from build123d import *

# Parameters (mm, degrees)
F1_DEPTH = 5
F2_W     = 5
F2_H     = 5
F3_DEPTH = 85
F4_W     = 2
F4_H     = 10
F5_DEPTH = 5
F6_DEPTH = 5
F7_R     = 1
F8_DEPTH = 10


with BuildPart() as f1:
    # F0 (on Top) → F1 (new body)
    with BuildSketch(Plane.XY):
        Polygon((3.1958913997, 17.8316862418), (3.1958913997, 29.6752474937), (-5.6755073997, 29.6752474937), (-5.6755073997, 17.4481306137), (-3.004598, 19.391063), (-2.590673, 19.643703), (-2.127576, 19.830687), (-1.639877, 19.938255), (-1.14109, 19.963425), (-0.645039, 19.905499), (-0.165471, 19.766083), (0.284322, 19.549041), align=None)
        with BuildLine():
            Line((44.778874, -6.695544), (3.1958913997, 17.8316862418))
            Line((3.1958913997, 17.8316862418), (3.1958913997, 16.96755))
            Line((3.1958913997, 16.96755), (-0.239810875, 16.96755))
            ThreePointArc((-0.239810875, 16.96755), (-1.239808, 15.967552875), (-2.239805125, 16.96755))
            Line((-2.239805125, 16.96755), (-5.6755073997, 16.96755))
            Line((-5.6755073997, 16.96755), (-5.6755073997, 17.4481306137))
            Line((-5.6755073997, 17.4481306137), (-44.778874, -10.997311))
            Line((-44.778874, -10.997311), (-44.506651, -11.416707))
            Line((-44.506651, -11.416707), (-44.230389, -11.833453))
            Line((-44.230389, -11.833453), (-43.950113, -12.24751))
            Line((-43.950113, -12.24751), (-43.66585, -12.65884))
            Line((-43.66585, -12.65884), (-43.377624, -13.067404))
            Line((-43.377624, -13.067404), (-43.085465, -13.473164))
            Line((-43.085465, -13.473164), (-42.789399, -13.876081))
            Line((-42.789399, -13.876081), (-42.489453, -14.276119))
            Line((-42.489453, -14.276119), (-42.185655, -14.673241))
            Line((-42.185655, -14.673241), (-41.878035, -15.067408))
            Line((-41.878035, -15.067408), (-41.56662, -15.458584))
            Line((-41.56662, -15.458584), (-41.25144, -15.846733))
            Line((-41.25144, -15.846733), (-40.932525, -16.231819))
            Line((-40.932525, -16.231819), (-40.609903, -16.613804))
            Line((-40.609903, -16.613804), (-40.283605, -16.992655))
            Line((-40.283605, -16.992655), (-39.953662, -17.368335))
            Line((-39.953662, -17.368335), (-39.620104, -17.74081))
            Line((-39.620104, -17.74081), (-39.282963, -18.110044))
            Line((-39.282963, -18.110044), (-38.942269, -18.476003))
            Line((-38.942269, -18.476003), (-38.598056, -18.838653))
            Line((-38.598056, -18.838653), (-38.250354, -19.19796))
            Line((-38.250354, -19.19796), (-37.899197, -19.553891))
            Line((-37.899197, -19.553891), (-37.544616, -19.906411))
            Line((-37.544616, -19.906411), (-37.486622, -19.963425))
            Line((-37.486622, -19.963425), (-33.507621, -18.914429))
            Line((-33.507621, -18.914429), (-33.877651, -18.578163))
            Line((-33.877651, -18.578163), (-34.244177, -18.23808))
            Line((-34.244177, -18.23808), (-34.60716, -17.894218))
            Line((-34.60716, -17.894218), (-34.966561, -17.546614))
            Line((-34.966561, -17.546614), (-35.322341, -17.195304))
            Line((-35.322341, -17.195304), (-35.674461, -16.840326))
            Line((-35.674461, -16.840326), (-36.022885, -16.481719))
            Line((-36.022885, -16.481719), (-36.367574, -16.119522))
            Line((-36.367574, -16.119522), (-36.708491, -15.753772))
            Line((-36.708491, -15.753772), (-37.045601, -15.384509))
            Line((-37.045601, -15.384509), (-37.378867, -15.011774))
            Line((-37.378867, -15.011774), (-37.708252, -14.635605))
            Line((-37.708252, -14.635605), (-38.033722, -14.256044))
            Line((-38.033722, -14.256044), (-38.355242, -13.87313))
            Line((-38.355242, -13.87313), (-38.672778, -13.486906))
            Line((-38.672778, -13.486906), (-38.986294, -13.097412))
            Line((-38.986294, -13.097412), (-39.295758, -12.704691))
            Line((-39.295758, -12.704691), (-39.601136, -12.308785))
            Line((-39.601136, -12.308785), (-39.902395, -11.909735))
            Line((-39.902395, -11.909735), (-40.199504, -11.507586))
            Line((-40.199504, -11.507586), (-40.262255, -11.421522))
            Line((-40.262255, -11.421522), (-3.665827, 15.200266))
            Line((-3.665827, 15.200266), (-3.339439, 14.822254))
            Line((-3.339439, 14.822254), (-2.954863, 14.503627))
            Line((-2.954863, 14.503627), (-2.522758, 14.253214))
            Line((-2.522758, 14.253214), (-2.055097, 14.077956))
            Line((-2.055097, 14.077956), (-1.564842, 13.982709))
            Line((-1.564842, 13.982709), (-1.06558, 13.970114))
            Line((-1.06558, 13.970114), (-0.571146, 14.040519))
            Line((-0.571146, 14.040519), (-0.095243, 14.191973))
            Line((-0.095243, 14.191973), (0.34894, 14.420279))
            Line((0.34894, 14.420279), (0.749093, 14.719109))
            Line((0.749093, 14.719109), (1.094126, 15.080183))
            Line((1.094126, 15.080183), (1.344177, 15.440914))
            Line((1.344177, 15.440914), (40.323708, -7.550701))
            Line((40.323708, -7.550701), (40.067458, -7.980043))
            Line((40.067458, -7.980043), (39.806774, -8.406706))
            Line((39.806774, -8.406706), (39.541683, -8.830645))
            Line((39.541683, -8.830645), (39.272214, -9.251815))
            Line((39.272214, -9.251815), (38.998395, -9.67017))
            Line((38.998395, -9.67017), (38.720256, -10.085665))
            Line((38.720256, -10.085665), (38.437827, -10.498257))
            Line((38.437827, -10.498257), (38.151138, -10.907899))
            Line((38.151138, -10.907899), (37.86022, -11.31455))
            Line((37.86022, -11.31455), (37.565104, -11.718164))
            Line((37.565104, -11.718164), (37.265821, -12.118698))
            Line((37.265821, -12.118698), (36.962405, -12.51611))
            Line((36.962405, -12.51611), (36.654888, -12.910357))
            Line((36.654888, -12.910357), (36.343302, -13.301397))
            Line((36.343302, -13.301397), (36.02768, -13.689187))
            Line((36.02768, -13.689187), (35.708058, -14.073686))
            Line((35.708058, -14.073686), (35.384469, -14.454852))
            Line((35.384469, -14.454852), (35.056948, -14.832646))
            Line((35.056948, -14.832646), (34.72553, -15.207025))
            Line((34.72553, -15.207025), (34.390251, -15.57795))
            Line((34.390251, -15.57795), (34.318334, -15.656515))
            Line((34.318334, -15.656515), (35.327871, -19.64571))
            Line((35.327871, -19.64571), (35.67992, -19.290661))
            Line((35.67992, -19.290661), (36.028522, -18.932227))
            Line((36.028522, -18.932227), (36.373644, -18.570442))
            Line((36.373644, -18.570442), (36.715254, -18.205338))
            Line((36.715254, -18.205338), (37.05332, -17.836951))
            Line((37.05332, -17.836951), (37.387811, -17.465314))
            Line((37.387811, -17.465314), (37.718695, -17.090462))
            Line((37.718695, -17.090462), (38.045942, -16.712431))
            Line((38.045942, -16.712431), (38.369521, -16.331256))
            Line((38.369521, -16.331256), (38.689401, -15.946971))
            Line((38.689401, -15.946971), (39.005553, -15.559614))
            Line((39.005553, -15.559614), (39.317948, -15.16922))
            Line((39.317948, -15.16922), (39.626556, -14.775825))
            Line((39.626556, -14.775825), (39.931348, -14.379467))
            Line((39.931348, -14.379467), (40.232296, -13.980182))
            Line((40.232296, -13.980182), (40.529372, -13.578008))
            Line((40.529372, -13.578008), (40.822549, -13.172983))
            Line((40.822549, -13.172983), (41.111797, -12.765143))
            Line((41.111797, -12.765143), (41.397092, -12.354527))
            Line((41.397092, -12.354527), (41.678405, -11.941174))
            Line((41.678405, -11.941174), (41.955712, -11.525122))
            Line((41.955712, -11.525122), (42.228985, -11.10641))
            Line((42.228985, -11.10641), (42.498199, -10.685077))
            Line((42.498199, -10.685077), (42.76333, -10.261162))
            Line((42.76333, -10.261162), (43.024353, -9.834706))
            Line((43.024353, -9.834706), (43.281242, -9.405747))
            Line((43.281242, -9.405747), (43.533975, -8.974325))
            Line((43.533975, -8.974325), (43.782527, -8.540482))
            Line((43.782527, -8.540482), (44.026875, -8.104258))
            Line((44.026875, -8.104258), (44.266997, -7.665692))
            Line((44.266997, -7.665692), (44.50287, -7.224827))
            Line((44.50287, -7.224827), (44.734473, -6.781704))
            Line((44.734473, -6.781704), (44.778874, -6.695544))
        make_face()
        with BuildLine():
            Line((3.1958913997, 16.96755), (3.1958913997, 17.8316862418))
            Line((3.1958913997, 17.8316862418), (0.284322, 19.549041))
            Line((0.284322, 19.549041), (-0.165471, 19.766083))
            Line((-0.165471, 19.766083), (-0.645039, 19.905499))
            Line((-0.645039, 19.905499), (-1.14109, 19.963425))
            Line((-1.14109, 19.963425), (-1.639877, 19.938255))
            Line((-1.639877, 19.938255), (-2.127576, 19.830687))
            Line((-2.127576, 19.830687), (-2.590673, 19.643703))
            Line((-2.590673, 19.643703), (-3.004598, 19.391063))
            Line((-3.004598, 19.391063), (-5.6755073997, 17.4481306137))
            Line((-5.6755073997, 17.4481306137), (-5.6755073997, 16.96755))
            Line((-5.6755073997, 16.96755), (-2.239805125, 16.96755))
            ThreePointArc((-2.239805125, 16.96755), (-1.239808, 17.967547125), (-0.239810875, 16.96755))
            Line((-0.239810875, 16.96755), (3.1958913997, 16.96755))
        make_face()
    extrude(amount=F1_DEPTH)

    # F2 (on face) → F3 (join)
    with BuildSketch(Plane(origin=(0, 29.6752474937, 0), x_dir=(-1, 0, 0), z_dir=(0, 1, 0))):
        with Locations((1.239808, 2.5)):
            Rectangle(F2_W, F2_H)
    extrude(amount=F3_DEPTH)

    # F4 (on face) → F5 (join)
    with BuildSketch(Plane.XY.offset(5)):
        with Locations((-4.739808, 109.6752474937)):
            Rectangle(F4_W, F4_H)
        with Locations((2.260192, 109.6752474937)):
            Rectangle(F4_W, F4_H)
    extrude(amount=-F5_DEPTH)

    # F4 (on face) → F6 (cut)
    with BuildSketch(Plane.XY.offset(5)):
        Polygon((-0.239808, 114.6752474937), (-2.239808, 114.6752474937), (-2.739808, 108.6752474937), (0.260192, 108.6752474937), align=None)
    extrude(amount=-F6_DEPTH, mode=Mode.SUBTRACT)

    # F7 (on face) → F8 (cut)
    with BuildSketch(Plane.YZ.offset(3.260192)):
        with Locations((121.0267286794, 2.5)):
            Circle(F7_R)
    extrude(amount=-F8_DEPTH, mode=Mode.SUBTRACT)


solid = f1.part
Verification items for the finished model (mm, model axes). A direction names the side the tool comes from. Coordinates: 2 decimals unless noted, no trailing zeros. Order: outer loops, then holes, each group sorted by start corner. A loop starts at its lowest first (then second) coordinate and runs counter-clockwise, first axis right, second up.
Item 1: Material ranges on L1, parallel to X at y = 18, z = 3.55; L2, parallel to X at y = 82, z = 4.35; L3, parallel to X at y = 11, z = 1.55, recorded low to high.
Filled in:
L1: x = -5.68 to 3.2
L2: x = -3.74 to 1.26
L3: x = -14.54 to -9.44, 8.87 to 14.78
Item 2: Section check B-B, the plane y = 25. Enter the section's corners in (x, z), then the cut area to 3 significant figures.
Filled in:
outline: (-5.68, 0) - (3.2, 0) - (3.2, 5) - (-5.68, 5) - close
area: 44.4 mm2
Item 3: Depth check by flat-ended pin: pin 1 (1.5 mm diameter, centred on y = 74, z = 3.5, fed in from +X); pin 2 (1.5 mm diameter, centred on y = 111.5, z = 2, fed in from -X); pin 3 (2 mm diameter, centred on y = 67, z = 1, fed in from -X); pin 4 (2.5 mm diameter, centred on x = -1.5, z = 1.5, fed in from +Y). Enter the tip coordinate at first touch or a pass-through.
Filled in:
pin 1: stops at x = 1.26
pin 2: stops at x = -5.74
pin 3: stops at x = -3.74
pin 4: stops at y = 114.68
Item 4: Release check for a two-part mould opening along X. For faces 4 (the face through (34.816, -17.623, 2.465)), 5 (the face through (0, 43, 0)), 6 (the face through (-2.486, 111.717, 2.535)), 7 (the face through (-24.953, 3.425, 2.465)) record: +X half, -X half, draft (parallel to the pull), parting line (faces both ways), or undercut.
Filled in:
face 4: undercut
face 5: draft
face 6: undercut
face 7: -X half
Item 5: Access from +Z, -Z, +X, -X, +Y, -Y to the whole of each face (thin tool, end or side, straight path). Record for faces 1 (the face through (1.26, 67, 2)), 2 (the face through (-35.525, -19.446, 2.465)), 3 (the face through (-22.22, 1.703, 2.465)).
Filled in:
face 1: +Z, -Z, +X
face 2: +Z, -Z, -Y
face 3: +Z, -Z
Item 6: Section check C-C, the plane x = -28. Enter the section's corners in (y, z).
Filled in:
outline: (-2.5, 0) - (1.21, 0) - (1.21, 5) - (-2.5, 5) - close
Item 7: Section check A-A, the plane y = 11. Enter the section's corners in (x, z), then the cut area to 3 significant figures.
Filled in:
outline: (-14.54, 0) - (-9.44, 0) - (-9.44, 5) - (-14.54, 5) - close; (8.87, 0) - (14.78, 0) - (14.78, 5) - (8.87, 5) - close
area: 55.0 mm2
